from build123d import *

# Parameters (mm, degrees)
F0_W     = 1212
F0_H     = 160
F1_DEPTH = 19
F2_R     = 12.5
F3_DEPTH = 12
F5_D     = 8
F5_DEPTH = 22
F5_TIP   = 2.4034424761


# Not quite as in the source:
# - a pattern or mirror of a feature is missing from the dataset's text; its kind, count and spacing are read off the source's solid


with BuildPart() as f1:
    # F0 (on Front) → F1 (new body)
    with BuildSketch(Plane.XZ):
        Rectangle(F0_W, F0_H)
    extrude(amount=F1_DEPTH)

    # F2 (on face) → F3 (cut)
    with BuildSketch(Plane.XZ.offset(19)):
        with Locations((-572.5, 0)):
            Circle(F2_R)
    f3 = extrude(amount=-F3_DEPTH, mode=Mode.SUBTRACT)

    # F3_copies: F3 across plane
    add(f3.mirror(Plane(origin=(0, 0, 0), x_dir=(0, 0, 1), z_dir=(1, 0, 0))), mode=Mode.SUBTRACT)

    # F5
    with Locations(Plane(origin=(-606, 0, 0), x_dir=(0, -1, 0), z_dir=(-1, 0, 0))):
        with Locations((12, 0)):
            f5 = Hole(F5_D / 2, depth=F5_DEPTH)
            with Locations((0, 0, -(F5_DEPTH + F5_TIP / 2))):  # 118° drill point
                Cone(0, F5_D / 2, F5_TIP, mode=Mode.SUBTRACT)

    # F5_copies: F5 across plane
    add(f5.mirror(Plane(origin=(3.5e-05, 0, 0), x_dir=(0, 0, 1), z_dir=(1, 0, 0))), mode=Mode.SUBTRACT)


solid = f1.part
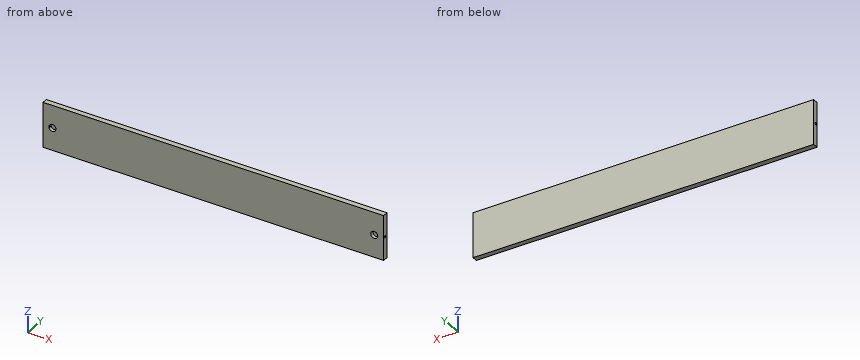
The model under review builds one solid part; all positions refer to its coordinate system, in mm. Coordinates: 2 decimals unless noted, no trailing zeros. Write each loop counter-clockwise with the first axis right and the second up, starting at its lowest first coordinate (ties: lowest second). Pieces come first, ordered by that corner, then holes. Notation, with made-up numbers: (-18, 42) - (17, 42) arc R19 ccw to (17, 79) - close; hole circle Ø11 at (-8.5, -33.5). An arc over 180 degrees is marked (long way). Answer as a JSON object with one key per item and string values. Group by question number.
1. To check wall thickness, follow probe 1 along X at (y, z) = (-16.5, 0); probe 2 along Y at (x, z) = (-595.5, 0); probe 3 along Z at (x, y) = (-572.5, -12). State the ranges of each line that lie inside material, in increasing order.
2. Clearance check with flat-ended pins moving along their axes: pin 1 Ø20 at (x, z) = (-578, 3.5) entering from -Y; pin 2 Ø5 at (y, z) = (-12, 0) entering from -X. State where each tip first meets the part, or that it passes through.
3. Add section A-A (x = -572.5). Give the boundary of the cut face in (y, z).
Findings:
{
 "1": {"probe 1": "-606 to -585, -560 to 560, 585 to 606", "probe 2": "-19 to -16, -8 to 0", "probe 3": "-80 to -12.5, 12.5 to 80"},
 "2": {"pin 1": "y = -19", "pin 2": "x = -560.25"},
 "3": {"outline": "(-19, -80) - (0, -80) - (0, 80) - (-19, 80) - (-19, 12.5) - (-7, 12.5) - (-7, -12.5) - (-19, -12.5) - close"}
}
